from build123d import *

# Parameters (mm, degrees)
SKETCH1_W           = 13.84
SKETCH1_H           = 17.13
BOSS_EXTRUDE1_DEPTH = 29.84
SKETCH2_R           = 1.5
CUT_EXTRUDE1_DEPTH  = 29.84
BOSS_EXTRUDE2_DEPTH = 1.4
FILLET1_R           = 2
FILLET2_R           = 1
SKETCH4_W           = 10.2
SKETCH4_H           = 1.4
CUT_EXTRUDE2_DEPTH  = 38.202618523
SKETCH5_R           = 6.25
SKETCH5_R_2         = 1.5
BOSS_EXTRUDE3_DEPTH = 26.84


with BuildPart() as part:
    # Sketch1 → Boss-Extrude1 (new body)
    with BuildSketch(Plane(origin=(0, 0, 0), x_dir=(0, 0, -1), z_dir=(1, 0, 0))):
        Rectangle(SKETCH1_W, SKETCH1_H)
    extrude(amount=BOSS_EXTRUDE1_DEPTH)

    # Sketch2 → Cut-Extrude1 (cut)
    with BuildSketch(Plane.ZY):
        Circle(SKETCH2_R)
    extrude(amount=-CUT_EXTRUDE1_DEPTH, mode=Mode.SUBTRACT)

    # Sketch3 → Boss-Extrude2 (add)
    # profile 1 of 2: a face of its own
    with BuildSketch(Plane.XZ.offset(8.565)):
        with BuildLine():
            Line((20.64, 9.455), (20.64, 6.92))
            Line((20.64, 6.92), (29.49, 6.92))
            Line((29.49, 6.92), (29.49, 9.455))
            ThreePointArc((29.49, 9.455), (28.281815472, 12.371815472), (25.365, 13.58))
            Line((25.365, 13.58), (24.765, 13.58))
            ThreePointArc((24.765, 13.58), (21.848184528, 12.371815472), (20.64, 9.455))
        make_face()
        with BuildLine():
            ThreePointArc((24.765, 7.58), (22.89, 9.455), (24.765, 11.33))
            Line((24.765, 11.33), (25.365, 11.33))
            ThreePointArc((25.365, 11.33), (27.24, 9.455), (25.365, 7.58))
            Line((25.365, 7.58), (24.765, 7.58))
        make_face(mode=Mode.SUBTRACT)
    # profile 2 of 2: a face of its own
    with BuildSketch(Plane.XZ.offset(8.565)):
        with BuildLine():
            Line((3.84, -6.92), (3.84, -9.455))
            ThreePointArc((3.84, -9.455), (5.048184528, -12.371815472), (7.965, -13.58))
            Line((7.965, -13.58), (8.565, -13.58))
            ThreePointArc((8.565, -13.58), (11.481815472, -12.371815472), (12.69, -9.455))
            Line((12.69, -9.455), (12.69, -6.92))
            Line((12.69, -6.92), (3.84, -6.92))
        make_face()
        with BuildLine():
            ThreePointArc((8.565, -7.58), (10.44, -9.455), (8.565, -11.33))
            Line((8.565, -11.33), (7.965, -11.33))
            ThreePointArc((7.965, -11.33), (6.09, -9.455), (7.965, -7.58))
            Line((7.965, -7.58), (8.565, -7.58))
        make_face(mode=Mode.SUBTRACT)
    extrude(amount=-BOSS_EXTRUDE2_DEPTH)

    # Fillet1
    fillet1_edges = [part.edges().sort_by_distance(p)[0] for p in [
        (0, -8.565, 0),
        (0, 8.565, 0),
    ]]
    fillet(fillet1_edges, radius=FILLET1_R)

    # Fillet2
    # the kernel refuses this fillet: 1 mm, written as the material it adds along each edge
    with BuildSketch(Plane(origin=(3.84, -8.565, -6.92), x_dir=(-1, 0, 0), z_dir=(0, 1, 0))) as fillet2_piece_1:
        with BuildLine():
            CenterArc((FILLET2_R, -FILLET2_R), FILLET2_R, 90, 90)
            Line((0, -FILLET2_R), (-FILLET2_R * 0.02, -FILLET2_R))
            Line((-FILLET2_R * 0.02, -FILLET2_R), (-FILLET2_R * 0.02, FILLET2_R * 0.02))
            Line((-FILLET2_R * 0.02, FILLET2_R * 0.02), (FILLET2_R, FILLET2_R * 0.02))
            Line((FILLET2_R, FILLET2_R * 0.02), (FILLET2_R, 0))
        make_face()
    extrude(amount=1.4)
    with BuildSketch(Plane(origin=(20.64, -8.565, 6.92), x_dir=(-1, 0, 0), z_dir=(0, 1, 0)), Plane(origin=(12.69, -8.565, -6.92), x_dir=(1, 0, 0), z_dir=(0, 1, 0))) as fillet2_piece_2:
        with BuildLine():
            CenterArc((FILLET2_R, FILLET2_R), FILLET2_R, 180, 90)
            Line((0, FILLET2_R), (-FILLET2_R * 0.02, FILLET2_R))
            Line((-FILLET2_R * 0.02, FILLET2_R), (-FILLET2_R * 0.02, -FILLET2_R * 0.02))
            Line((-FILLET2_R * 0.02, -FILLET2_R * 0.02), (FILLET2_R, -FILLET2_R * 0.02))
            Line((FILLET2_R, -FILLET2_R * 0.02), (FILLET2_R, 0))
        make_face()
    extrude(amount=1.4)
    with BuildSketch(Plane(origin=(29.49, -8.565, 6.92), x_dir=(1, 0, 0), z_dir=(0, 1, 0))) as fillet2_piece_3:
        with BuildLine():
            CenterArc((1, -0.759934208), FILLET2_R, 130.541601874, 49.458398126)
            Line((0, -0.759934208), (-0.02, -0.759934208))
            Line((-0.02, -0.759934208), (-0.02, 0))
            Line((-0.02, 0), (0, 0.02))
            ThreePointArc((0, 0.02), (0.175, 0.02), (0.337, 0.015198684))
            Line((0.337, 0.015198684), (0.35, 0))
        make_face()
    extrude(amount=1.4)

    # Sketch4 → Cut-Extrude2 (cut, through all)
    with BuildSketch(Plane.XY.offset(6.92)):
        with BuildLine():
            Line((18.14, -7.065), (18.14, -5.665))
            Line((18.14, -5.665), (28.34, -5.665))
            Line((28.34, -5.665), (28.34, 7.065))
            Line((28.34, 7.065), (2, 7.065))
            ThreePointArc((2, 7.065), (1.646446609, 6.918553391), (1.5, 6.565))
            Line((1.5, 6.565), (1.5, -6.565))
            ThreePointArc((1.5, -6.565), (1.646446609, -6.918553391), (2, -7.065))
            Line((2, -7.065), (18.14, -7.065))
        make_face()
        with Locations((23.24, -6.365)):
            Rectangle(SKETCH4_W, SKETCH4_H)
    extrude(amount=-CUT_EXTRUDE2_DEPTH, mode=Mode.SUBTRACT)

    # Sketch5 → Boss-Extrude3 (add)
    with BuildSketch(Plane(origin=(1.5, 0, 0), x_dir=(0, 0, -1), z_dir=(1, 0, 0))):
        with Locations(Location((0, 0, 0), (0, 0, 270))):
            Circle(SKETCH5_R)
        with Locations(Location((0, 0, 0), (0, 0, 180))):
            Circle(SKETCH5_R_2, mode=Mode.SUBTRACT)
    extrude(amount=BOSS_EXTRUDE3_DEPTH)


solid = part.part
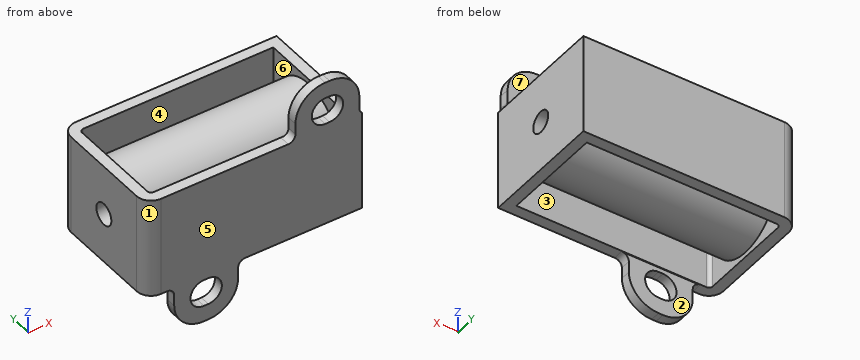
Could you check a few things on this model? Use its own coordinates, in mm. Face numbers are marked on the shaded views. A direction names the side the tool comes from. Coordinates: 2 decimals unless noted, no trailing zeros. Loops run counter-clockwise (first coordinate to the right, second up) from the corner with the lowest first, then second, coordinate; pieces in that order, holes last. Notation, with made-up numbers: (67, 0) -> (99, 0) arc R23 cw to (99, 10) -> close; hole circle Ø5 at (19.25, 3). An arc over 180 degrees is marked (long way). Answer in a Markdown table with one row per item.
(1) Will these pins go through, and if not, where does the flat tip stop? pin 1 Ø5.5 at (x, z) = (8, -12) entering from +Y (3 decimals); pin 2 Ø0.7 at (y, z) = (-7.5, -9) entering from +X; pin 3 Ø2 at (x, y) = (7.5, -6) entering from -Z; pin 4 Ø1.8 at (y, z) = (0, 0) entering from -X.
Results found:
| item | result |
|---|---|
| pin 1 | stops at y = -7.165 |
| pin 2 | stops at x = 12.69 |
| pin 3 | stops at z = -3.75 |
| pin 4 | passes through |
(2) Thinking about a two-plate mould opening in Y: for the marked faces 1, 2, 3 and 4, which applies, released by +Y, released by -Y, zero draft, split by the parting line, or undercut?
Results found:
| item | result |
|---|---|
| face 1 | released by -Y |
| face 2 | released by +Y |
| face 3 | undercut |
| face 4 | undercut |
(3) Imagine slicing it at A-A (z = 0). List the corners of the cut face in (x, y) for me (3 decimals).
Results found:
| item | result |
|---|---|
| outline | (0, -6.565) arc R2 ccw to (2, -8.565) -> (29.84, -8.565) -> (29.84, -1.5) -> (0, -1.5) -> close; (0, 1.5) -> (29.84, 1.5) -> (29.84, 8.565) -> (2, 8.565) arc R2 ccw to (0, 6.565) -> close; hole (1.5, -6.565) arc R0.5 ccw to (2, -7.065) -> (28.34, -7.065) -> (28.34, -6.25) -> (1.5, -6.25) -> close; hole (1.5, 6.25) -> (28.34, 6.25) -> (28.34, 7.065) -> (2, 7.065) arc R0.5 ccw to (1.5, 6.565) -> close |
(4) For the marked faces 5, 6 and 7, which set-ups out of +Z, -Z, +X, -X, +Y, -Y let a thin tool reach every point of the face, with its end or its side?
Results found:
| item | result |
|---|---|
| face 5 | +Z, -Z, +X, -X, -Y |
| face 6 | none |
| face 7 | +Z, +X, -X, +Y |
(5) Imagine slicing it at B-B (x = 5.5). List the corners of the cut face in (y, z) for me (3 decimals), plus the area to 3 significant figures.
Results found:
| item | result |
|---|---|
| outline | (-8.565, -12.762) -> (-7.165, -12.762) -> (-7.165, -6.92) -> (-7.065, -6.92) -> (-7.065, 6.92) -> (-8.565, 6.92) -> close; circle Ø12.5 at (0, 0); (7.065, -6.92) -> (8.565, -6.92) -> (8.565, 6.92) -> (7.065, 6.92) -> close; hole circle Ø3 at (0, 0) |
| area | 165 mm^2 |
(6) Imagine slicing it at C-C (y = 0). List the corners of the cut face in (x, z) for me.
Results found:
| item | result |
|---|---|
| outline | (0, -6.92) -> (1.5, -6.92) -> (1.5, -6.25) -> (28.34, -6.25) -> (28.34, -6.92) -> (29.84, -6.92) -> (29.84, -1.5) -> (0, -1.5) -> close; (0, 1.5) -> (29.84, 1.5) -> (29.84, 6.92) -> (28.34, 6.92) -> (28.34, 6.25) -> (1.5, 6.25) -> (1.5, 6.92) -> (0, 6.92) -> close |
(7) Imagine slicing it at D-D (z = 10.75). List the corners of the cut face in (x, y) for me (3 decimals), plus the area to 3 significant figures.
Results found:
| item | result |
|---|---|
| outline | (20.849, -8.565) -> (23.409, -8.565) -> (23.409, -7.165) -> (20.849, -7.165) -> close; (26.721, -8.565) -> (29.281, -8.565) -> (29.281, -7.165) -> (26.721, -7.165) -> close |
| area | 7.17 mm^2 |
(8) If I drill on probe 1 along X at (y, z) = (-6.25, 1); probe 2 along Y at (x, z) = (2, 6.75) (3 decimals); probe 3 along Y at (x, z) = (20.5, -4) (3 decimals), over which ranges is the centre line in solid material (lowest first)?
Results found:
| item | result |
|---|---|
| probe 1 | x = 0 to 1.5, 28.34 to 29.84 |
| probe 2 | y = -8.565 to -7.065, 7.065 to 8.565 |
| probe 3 | y = -8.565 to -7.065, -4.802 to 4.802, 7.065 to 8.565 |
